Can you work these out from the model? Positions are in its coordinate system, mm. A direction names the side the tool comes from. Give positions to 0.01 mm unless a question says otherwise; leave off trailing zeros. Order: outer loops, then holes, each group sorted by start corner. A loop starts at its lowest first (then second) coordinate and runs counter-clockwise, first axis right, second up. Notation, with made-up numbers: M -32,-37.5 L 3,-37.5 A7 ccw 3,-29.5 Z; hole C -28.5,29 d2. An arc over 180 degrees is marked long. Answer as a JSON object with one key per item and string values.
```python
from build123d import *

# Parameters (mm, degrees)
SKETCH_W             = 70
SKETCH_H             = 140
PAD_DEPTH            = 10
FILLET_R             = 3
FILLET001_R          = 3
SKETCH001_W          = 10
SKETCH001_H          = 10
POCKET_DEPTH         = 10.001
POCKET001_DEPTH      = 5
FILLET002_R          = 3
FILLET003_R          = 3
BODY_PLACEMENT_ANGLE = 90


with BuildPart() as part:
    # Sketch → Pad (new body)
    with BuildSketch(Plane.YZ):
        Rectangle(SKETCH_W, SKETCH_H)
    extrude(amount=PAD_DEPTH)

    # Fillet
    fillet_edges = [part.edges().sort_by_distance(p)[0] for p in [
        (10, 0, 70),
    ]]
    fillet(fillet_edges, radius=FILLET_R)

    # Fillet001
    fillet001_edges = [part.edges().sort_by_distance(p)[0] for p in [
        (10, 0, -70),
    ]]
    fillet(fillet001_edges, radius=FILLET001_R)

    # Sketch001 (on Face7 of Fillet001) → Pocket (cut, through all)
    with BuildSketch(Plane(origin=(0, 0, 0), x_dir=(0, 1, 0), z_dir=(-1, 0, 0))):
        with Locations((-20, 65)):
            Rectangle(SKETCH001_W, SKETCH001_H)
        with Locations((0, 65)):
            Rectangle(SKETCH001_W, SKETCH001_H)
        with Locations((20, 65)):
            Rectangle(SKETCH001_W, SKETCH001_H)
        with Locations((-20, -65)):
            Rectangle(SKETCH001_W, SKETCH001_H)
        with Locations((0, -65)):
            Rectangle(SKETCH001_W, SKETCH001_H)
        with Locations((20, -65)):
            Rectangle(SKETCH001_W, SKETCH001_H)
    extrude(amount=-POCKET_DEPTH, mode=Mode.SUBTRACT)

    # Sketch002 (on Face7 of Pocket) → Pocket001 (cut)
    with BuildSketch(Plane(origin=(0, 0, 0), x_dir=(0, 1, 0), z_dir=(-1, 0, 0))):
        with BuildLine():
            ThreePointArc((25, -65), (27.5, -67.5), (30, -65))
            Line((30, -65), (30, 65))
            ThreePointArc((30, 65), (27.5, 67.5), (25, 65))
            Line((25, -65), (25, 65))
        make_face()
        with BuildLine():
            ThreePointArc((-30, -70), (-27.5, -72.5), (-25, -70))
            Line((-25, -70), (-25, 65))
            ThreePointArc((-25, 65), (-27.5, 67.5), (-30, 65))
            Line((-30, -70), (-30, 65))
        make_face()
    extrude(amount=-POCKET001_DEPTH, mode=Mode.SUBTRACT)

    # Fillet002
    fillet002_edges = [part.edges().sort_by_distance(p)[0] for p in [
        (10, -35, 0),
    ]]
    fillet(fillet002_edges, radius=FILLET002_R)

    # Fillet003
    fillet003_edges = [part.edges().sort_by_distance(p)[0] for p in [
        (10, 35, 0),
    ]]
    fillet(fillet003_edges, radius=FILLET003_R)


with BuildPart() as part_1:
    # Body placement: moved
    add(part.part.rotate(Axis((0, 0, 0), (0, 1, 0)), BODY_PLACEMENT_ANGLE))


with BuildPart() as part_2:
    # Clone placement: moved
    add(part_1.part.moved(Location((70, 35, 0))))


solid = part_2.part
```
1) I want a section at D-D on y = 38.5. Write out the boundary of the cut face in (x, z).
Results found:
{"outline": "M 10,-10 L 130,-10 L 130,0 L 10,0 Z"}
2) For faces 5 (the face through (139.14, 69.1, -3.45)), 6 (the face through (136, 60, -6)), 7 (the face through (10, 35, -5)), which set-ups out of +Z, -Z, +X, -X, +Y, -Y let a thin tool reach every point of the face, with its end or its side?
Results found:
{"face 5": "+Z, -Z, +X, +Y", "face 6": "+Z, -Z, +X", "face 7": "+Z, -Z, -X"}
3) I need wall thicknesses on L1, parallel to Y at x = 71.5, z = -3; L2, parallel to X at y = 12.5, z = -3.75; L3, parallel to Z at x = 29, y = 7. Which ranges of each line are inside material? Lowest first, please.
Results found:
{"L1": "y = 0 to 5, 10 to 60, 65 to 70", "L2": "x = 10 to 130", "L3": "z = -10 to -5"}
4) I'm going to push flat-ended pins straight in: pin 1 Ø8 at (x, y) = (24, 60.5) entering from +Z; pin 2 Ø1 at (y, z) = (35.5, -7) entering from +X; pin 3 Ø1 at (y, z) = (32, -4.5) entering from -X. Where does each tip first touch, or does it pass through?
Results found:
{"pin 1": "stops at z = 0", "pin 2": "stops at x = 130", "pin 3": "stops at x = 10"}
5) I want a section at B-B on y = 62.5. Write out the boundary of the cut face in (x, z).
Results found:
{"outline": "M 0,-7 A3 ccw 3,-10 L 137,-10 A3 ccw 140,-7 L 140,0 L 137.5,0 L 137.5,-5 L 2.5,-5 L 2.5,0 L 0,0 Z"}
6) I want a section at A-A on x = 109. Write out the boundary of the cut face in (y, z), and give its area (3 significant figures).
Results found:
{"outline": "M 0,-7 A3 ccw 3,-10 L 67,-10 A3 ccw 70,-7 L 70,0 L 65,0 L 65,-5 L 60,-5 L 60,0 L 10,0 L 10,-5 L 5,-5 L 5,0 L 0,0 Z", "area": "646 mm²"}
7) I want a section at C-C on y = 7.5. Write out the boundary of the cut face in (x, z), and give its area (3 significant figures).
Results found:
{"outline": "M 0,-7 A3 ccw 3,-10 L 137,-10 A3 ccw 140,-7 L 140,-5 L 2.5,-5 L 2.5,0 L 0,0 Z", "area": "709 mm²"}
8) Thinking about a two-plate mould opening in Y: for faces 1 (the face through (0.9, 25.07, -9.14)), 2 (the face through (10, 15, -5)), 3 (the face through (0.9, 0.86, -3.55)), 4 (the face through (135, 20, -5)), which applies, pulls with the +Y half, pulls with the -Y half, needs draft (parallel to the pull), parting line crosses it, or undercut?
Results found:
{"face 1": "needs draft", "face 2": "undercut", "face 3": "pulls with the -Y half", "face 4": "undercut"}
